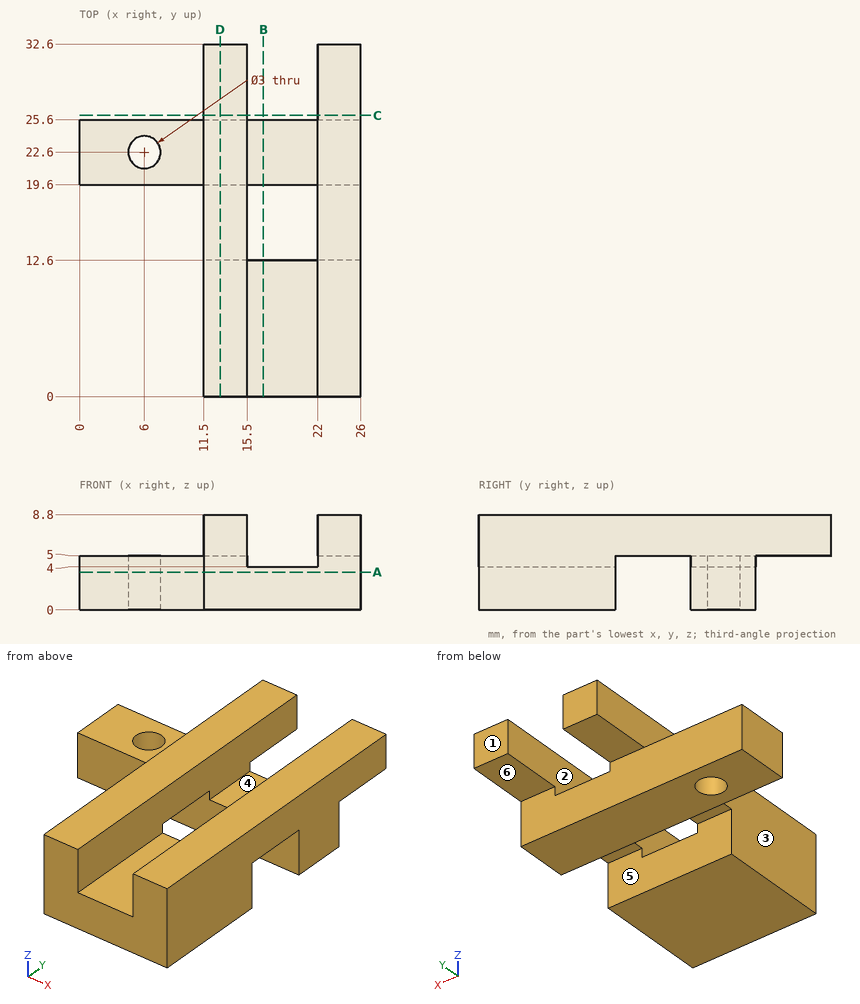
Verification items for this drawing (mm, ordinates from the low corner). A direction names the side the tool comes from. Coordinates: 2 decimals unless noted, no trailing zeros. Order: outer loops, then holes, each group sorted by start corner. A loop starts at its lowest first (then second) coordinate and runs counter-clockwise, first axis right, second up. Notation, with made-up numbers: (-27.5, 52.5) -> (8.5, 52.5) arc R18 cw to (8.5, 74.5) -> close; hole circle Ø2 at (50.5, -27). An arc over 180 degrees is marked (long way). Put each result on its own line as item: value. Start each with the question number.
1. Access from +Z, -Z, +X, -X, +Y, -Y to the whole of each face (thin tool, end or side, straight path). Record for the marked faces 4, 5 and 6.
2. Mould release check, pull along X, two halves, no side actions. Record for the marked faces 1, 2 and 3: released by +X, released by -X, zero draft, split by the parting line, or undercut.
3. Cross-section at C-C, the plane y = 26. Record the boundary of the cut face in (x, z).
4. Material ranges on L1, parallel to Y at x = 6, z = 3.6; L2, parallel to Y at x = 24, z = 3; L3, parallel to X at y = 28, z = 5.75, recorded low to high. Write a range as [from, to].
5. Cross-section at D-D, the plane x = 13. Record the boundary of the cut face in (y, z).
6. Go/stop test with flat-tipped pins: pin 1 Ø2 at (x, y) = (23.5, 17.5) entering from -Z; pin 2 Ø1.5 at (x, z) = (16.5, 2) entering from +Y; pin 3 Ø3 at (x, y) = (19.5, 23.5) entering from +Z; pin 4 Ø2.5 at (x, y) = (6, 22.6) entering from -Z. Record where each tip stops, or that it passes through.
7. Cross-section at B-B, the plane x = 17. Record the boundary of the cut face in (y, z), then the cut area to 3 significant figures.
8. Cross-section at A-A, the plane z = 3.5. Record the boundary of the cut face in (x, y).
Computed:
1. face 4: +Z, +Y, -Y
1. face 5: -Z, +X, -X
1. face 6: -Z, +X, -X, +Y
2. face 1: zero draft
2. face 2: undercut
2. face 3: released by -X
3. outline: (11.5, 5) -> (15.5, 5) -> (15.5, 8.8) -> (11.5, 8.8) -> close; (22, 5) -> (26, 5) -> (26, 8.8) -> (22, 8.8) -> close
4. L1: [19.6, 21.1], [24.1, 25.6]
4. L2: [0, 12.6], [19.6, 25.6]
4. L3: [11.5, 15.5], [22, 26]
5. outline: (0, 0) -> (12.6, 0) -> (12.6, 5) -> (19.6, 5) -> (19.6, 0) -> (25.6, 0) -> (25.6, 5) -> (32.6, 5) -> (32.6, 8.8) -> (0, 8.8) -> close
6. pin 1: z = 5
6. pin 2: y = 25.6
6. pin 3: z = 4
6. pin 4: through
7. outline: (0, 0) -> (12.6, 0) -> (12.6, 4) -> (0, 4) -> close; (19.6, 0) -> (25.6, 0) -> (25.6, 4) -> (19.6, 4) -> close
7. area: 74.4 mm2
8. outline: (0, 19.6) -> (26, 19.6) -> (26, 25.6) -> (0, 25.6) -> close; (11.5, 0) -> (26, 0) -> (26, 12.6) -> (11.5, 12.6) -> close; hole circle Ø3 at (6, 22.6)
